Here's how the part is built. I have some questions about the finished solid (model axes, mm). Face numbers are marked on the shaded views. A direction names the side the tool comes from. Give positions to 0.01 mm unless a question says otherwise; leave off trailing zeros. Write each loop counter-clockwise with the first axis right and the second up, starting at its lowest first coordinate (ties: lowest second). Pieces come first, ordered by that corner, then holes. Notation, with made-up numbers: (59.5, 34) - (102.5, 34) arc R31 cw to (102.5, 64) - close; hole circle Ø4 at (-22.75, 28). An arc over 180 degrees is marked (long way). Use a Markdown table: item, result.
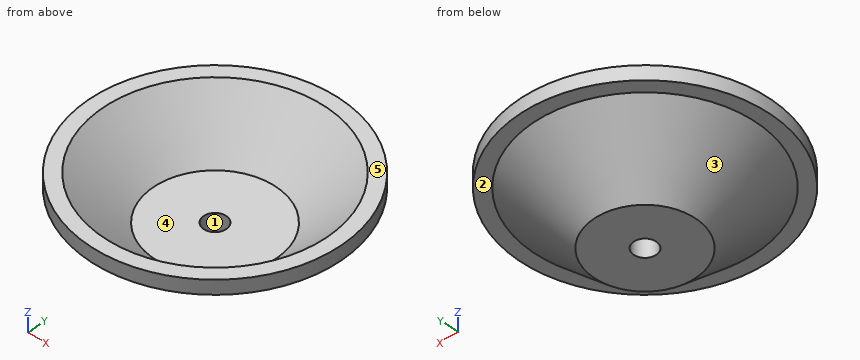
Solid Edge part; units mm, degrees
sketch "Sketch1" plane through (0, 0, 0) normal (0, -1, 0) x (1, 0, 0)
  line L0 (5, 24.31) -> (5, 32.81)
  line L1 (5, 32.81) -> (26.6959, 32.76)
  line L2 (44.4748, 49.3562) -> (26.6959, 32.76)
  line L3 (49.4748, 49.3562) -> (44.4748, 49.3562)
  line L4 (49.4748, 44.3562) -> (49.4748, 49.3562)
  line L5 (44.4748, 44.3562) -> (49.4748, 44.3562)
  line L6 (23, 24.31) -> (44.4748, 44.3562)
  line L7 (5, 24.31) -> (23, 24.31)
revolve "RevolvedProtrusion1" add sketch "Sketch1" angle 360 about axis through (5, 0, 15.0377) along (0, 0, 1)
hole "Hole1" at (5, 0, 32.81) direction (0, 0, -1) diameter 8 end through all
Item 1: If we section it at C-C, the plane z = 47.5: Write out the boundary of the cut face in (x, y), plus the area to 3 significant figures.
Values:
| item | result |
|---|---|
| outline | circle Ø88.95 at (5, 0); hole circle Ø74.97 at (5, 0) |
| area | 1,800 mm2 |
Item 2: For the marked faces 1 and 2, which set-ups out of +Z, -Z, +X, -X, +Y, -Y let a thin tool reach every point of the face, with its end or its side?
Values:
| item | result |
|---|---|
| face 1 | +Z, -Z |
| face 2 | -Z |
Item 3: If we section it at A-A, the plane y = 0: Write out the boundary of the cut face in (x, z), plus the area to 3 significant figures.
Values:
| item | result |
|---|---|
| outline | (-39.47, 44.36) - (-34.47, 44.36) - (-13, 24.31) - (1, 24.31) - (1, 32.8) - (-16.7, 32.76) - (-34.47, 49.36) - (-39.47, 49.36) - close; (9, 24.31) - (23, 24.31) - (44.47, 44.36) - (49.47, 44.36) - (49.47, 49.36) - (44.47, 49.36) - (26.7, 32.76) - (9, 32.8) - close |
| area | 515 mm2 |
Item 4: If we section it at B-B, the plane x = 5: Write out the boundary of the cut face in (y, z).
Values:
| item | result |
|---|---|
| outline | (-44.47, 44.36) - (-39.47, 44.36) - (-18, 24.31) - (-4, 24.31) - (-4, 32.8) - (-21.7, 32.76) - (-39.47, 49.36) - (-44.47, 49.36) - close; (4, 24.31) - (18, 24.31) - (39.47, 44.36) - (44.47, 44.36) - (44.47, 49.36) - (39.47, 49.36) - (21.7, 32.76) - (4, 32.8) - close |
Item 5: If we section it at D-D, the plane z = 36.75: Write out the boundary of the cut face in (x, y).
Values:
| item | result |
|---|---|
| outline | circle Ø62.65 at (5, 0); hole circle Ø51.94 at (5, 0) |
Item 6: I need wall thicknesses on line 1 along Z through (x, y) = (27, -34.5); line 2 along Y through (x, z) = (10.5, 37.25); line 3 along Z through (x, y) = (13, -5.5). Which ranges of each line are inside material? Lowest first, please. Write a range as [from, to].
Values:
| item | result |
|---|---|
| line 1 | z = [44.36, 49.36] |
| line 2 | y = [-31.38, -25.93], [25.93, 31.38] |
| line 3 | z = [24.31, 32.79] |
Item 7: Thinking about a two-plate mould opening in Y: for the marked faces 3, 4 and 5, which applies, +Y half, -Y half, draft (parallel to the pull), parting line (faces both ways), or undercut?
Values:
| item | result |
|---|---|
| face 3 | parting line |
| face 4 | undercut |
| face 5 | draft |
Item 8: Will these pins go through, and if not, where does the flat tip stop? pin 1 Ø1 at (y, z) = (-27, 46.5) entering from +X; pin 2 Ø2 at (y, z) = (-17, 29.5) entering from -X; pin 3 Ø1.5 at (x, y) = (17.5, 7) entering from +Z.
Values:
| item | result |
|---|---|
| pin 1 | stops at x = 40.72 |
| pin 2 | stops at x = -13.1 |
| pin 3 | stops at z = 32.78 |
